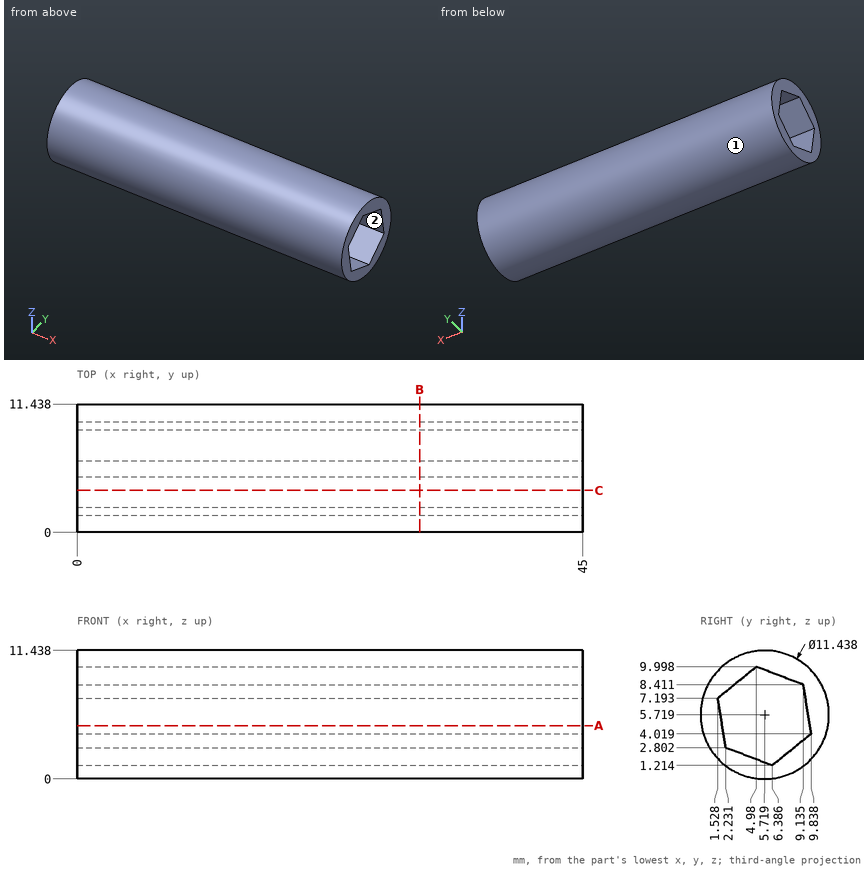
Design review of the part shown in the three views and the two pictorial views. Dimensions are in mm from the part's minimum x, y and z. Give positions to 0.01 mm unless a question says otherwise; leave off trailing zeros. Loops run counter-clockwise (first coordinate to the right, second up) from the corner with the lowest first, then second, coordinate; pieces in that order, holes last. Notation, with made-up numbers: (41.25, 17.25) -> (50.25, 17.25) arc R11 cw to (50.25, 33.25) -> close; hole circle Ø4 at (42.25, -11.75). An arc over 180 degrees is marked (long way). Put each result on its own line as item: value. Start each with the question number.
1. We need section A-A on z = 4.75. State the section outline as (x, y) points (1 decimal), then the cut area to 3 significant figures.
2. Mouldability with a two-part tool opening along Y and no side actions: class the marked faces 1 and 2 as released by +Y, released by -Y, zero draft, split by the parting line, or undercut.
3. We need section B-B on x = 30.5. State the section outline as (y, z) points (1 decimal).
4. We need section C-C on y = 3.75. State the section outline as (x, z) points.
5. Wall thickness on probe 1 along Z at (x, y) = (14.5, 5.5) (1 decimal); probe 2 along Y at (x, z) = (22, 4) (1 decimal); probe 3 along Y at (x, z) = (31.5, 7) (1 decimal): over which ranges is each line inside the solid? List them lowest first.
6. Clearance check with flat-ended pins moving along their axes: P1, Ø2, axis at x = 17.5, y = 6.5, coming from the +Z side; P2, Ø1, axis at x = 32.5, z = 3, coming from the +Y side; P3, Ø1, axis at x = 16.5, z = 9, coming from the +Y side. State where each tip first meets the part, or that it passes through.
Determined:
1. outline: (0, 0.1) -> (45, 0.1) -> (45, 1.9) -> (0, 1.9) -> close; (0, 9.7) -> (45, 9.7) -> (45, 11.4) -> (0, 11.4) -> close
1. area: 156 mm^2
2. face 1: split by the parting line
2. face 2: undercut
3. outline: circle Ø11.4 at (5.7, 5.7); hole (1.5, 7.2) -> (2.2, 2.8) -> (6.4, 1.2) -> (9.8, 4) -> (9.1, 8.4) -> (5, 10) -> close
4. outline: (0, 0.35) -> (45, 0.35) -> (45, 2.22) -> (0, 2.22) -> close; (0, 9) -> (45, 9) -> (45, 11.09) -> (0, 11.09) -> close
5. probe 1: 0 to 1.6, 9.8 to 11.4
5. probe 2: 0.3 to 2, 9.8 to 11.2
5. probe 3: 0.1 to 1.6, 9.4 to 11.3
6. P1: z = 11.44
6. P2: y = 10.99
6. P3: y = 10.72
